Can you work these out from the drawing? Everything is in mm from the part's minimum corner. Coordinates: 2 decimals unless noted, no trailing zeros. Order: outer loops, then holes, each group sorted by start corner. A loop starts at its lowest first (then second) coordinate and runs counter-clockwise, first axis right, second up. Notation, with made-up numbers: (30, 26) -> (40, 26) arc R23 ccw to (40, 52) -> close; hole circle Ø10 at (-19, 6.25). An arc over 180 degrees is marked (long way). Answer in a Markdown table with one row per item.
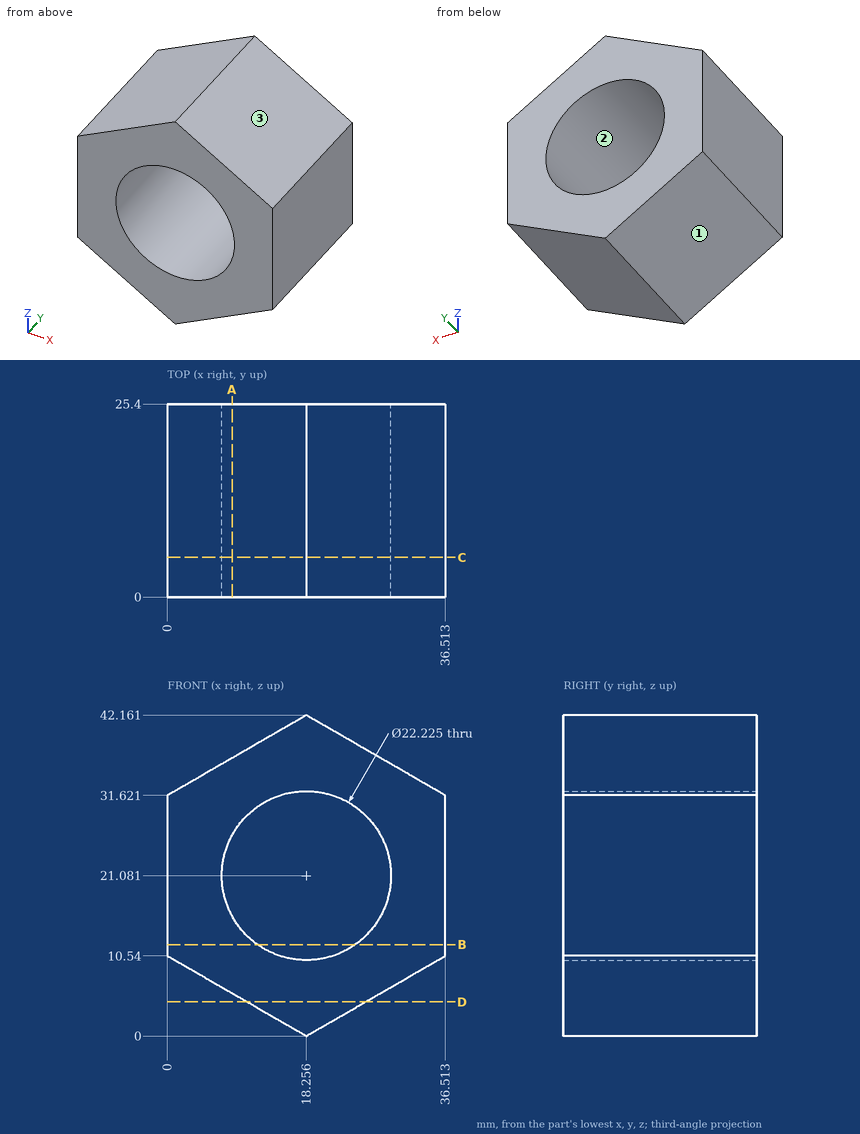
(1) Suppose I cut it at D-D (z = 4.5). Please give me the cut outline in (x, y), and give its area (3 significant figures).
Response values:
| item | result |
|---|---|
| outline | (10.46, 0) -> (26.05, 0) -> (26.05, 25.4) -> (10.46, 25.4) -> close |
| area | 396 mm2 |
(2) I need wall thicknesses on line 1 (X direction, y = 1, z = 21) (1 decimal); line 2 (X direction, y = 21.25, z = 11) (1 decimal); line 3 (Z direction, x = 22, y = 5.5) (1 decimal). Which ranges of each line are inside material? Lowest first, please. Write a range as [from, to].
Response values:
| item | result |
|---|---|
| line 1 | [0, 7.1], [29.4, 36.5] |
| line 2 | [0, 13.6], [22.9, 36.5] |
| line 3 | [2.2, 10.6], [31.5, 40] |
(3) Suppose I cut it at C-C (y = 5.25). Please give me the cut outline in (x, z) (1 decimal).
Response values:
| item | result |
|---|---|
| outline | (0, 10.5) -> (18.3, 0) -> (36.5, 10.5) -> (36.5, 31.6) -> (18.3, 42.2) -> (0, 31.6) -> close; hole circle Ø22.2 at (18.3, 21.1) |
(4) Will these pins go through, and if not, where does the flat tip stop? pin 1 Ø1.5 at (x, y) = (32.5, 10) entering from +Z; pin 2 Ø2 at (y, z) = (12, 37.5) entering from +X.
Response values:
| item | result |
|---|---|
| pin 1 | z = 34.37 |
| pin 2 | x = 28.06 |
(5) We'd pull the mould along X, two halves only. Please class the marked faces 1, 2 and 3: +X half, -X half, draft (parallel to the pull), parting line (faces both ways), or undercut.
Response values:
| item | result |
|---|---|
| face 1 | -X half |
| face 2 | undercut |
| face 3 | +X half |
(6) Suppose I cut it at B-B (z = 12). Please give me the cut outline in (x, y).
Response values:
| item | result |
|---|---|
| outline | (0, 0) -> (11.85, 0) -> (11.85, 25.4) -> (0, 25.4) -> close; (24.66, 0) -> (36.51, 0) -> (36.51, 25.4) -> (24.66, 25.4) -> close |
(7) Suppose I cut it at A-A (x = 8.5). Please give me the cut outline in (y, z).
Response values:
| item | result |
|---|---|
| outline | (0, 5.63) -> (25.4, 5.63) -> (25.4, 15.76) -> (0, 15.76) -> close; (0, 26.4) -> (25.4, 26.4) -> (25.4, 36.53) -> (0, 36.53) -> close |
